Build history of the part. All positions in model axes, mm. Give positions to 0.01 mm unless a question says otherwise; leave off trailing zeros. Order: outer loops, then holes, each group sorted by start corner. A loop starts at its lowest first (then second) coordinate and runs counter-clockwise, first axis right, second up. Notation, with made-up numbers: M -35.5,-6 L -9.5,-6 A9 cw -9.5,1 Z; hole C -10,23 d11. An arc over 180 degrees is marked long. One line per item, written item: value.
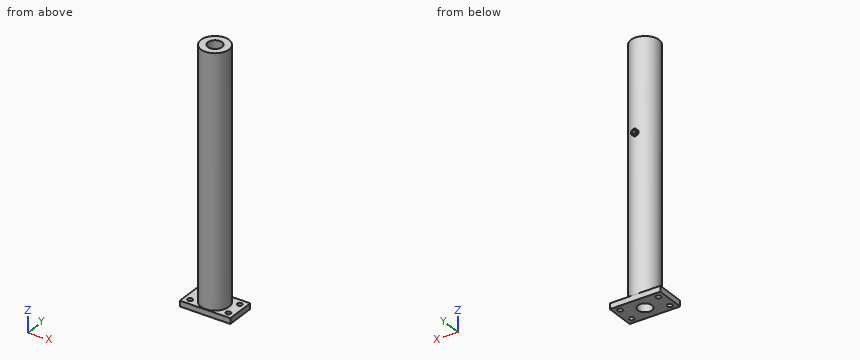
Autodesk Fusion 360 part; units mm, degrees
sketch "Sketch1" plane through (0, 0, 0) normal (0, 0, 1) x (1, 0, 0)
  circle A0 centre (0, 0) radius 6.375
  circle A1 centre (0, 0) radius 12.5
  dimension "d1" = 25
  dimension "d2" = 12.75
extrude "Extrude1" add sketch "Sketch1" along normal blind 225 contours A0 | A1
extrude "Extrude19" cut sketch "Sketch1" along normal up to surface (225 mm away) contours A0
sketch "Sketch22" plane through (0, 0, 0) normal (0, 0, 1) x (1, 0, 0)
  line L0 (22.5, 13) -> (-22.5, 13)
  line L1 (-22.5, 13) -> (-22.5, -13)
  line L2 (-22.5, -13) -> (22.5, -13)
  line L3 (22.5, -13) -> (22.5, 13)
  circle A0 centre (0, 0) radius 6.375 construction
  circle A1 centre (0, 0) radius 12.5 construction
  line L4 (0, 0) -> (22.5, 0) construction
  line L5 (0, 0) -> (-22.5, 0) construction
  circle A2 centre (0, 0) radius 12.5
  circle A3 centre (17, 7.5) radius 2.25
  circle A4 centre (-17, 7.5) radius 2.25
  circle A5 centre (-17, -7.5) radius 2.25
  circle A6 centre (17, -7.5) radius 2.25
  point P0 (12.5, 0)
  point P1 (-12.5, 0)
  dimension "d150" = 10
  dimension "d151" = 10
  dimension "d152" = 13
  dimension "d155" = 4.5
  dimension "d156" = 17
  dimension "d157" = 17
  dimension "d158" = 17
  dimension "d159" = 17
  dimension "d160" = 4.5
  dimension "d161" = 4.5
  dimension "d162" = 4.5
  dimension "d163" = 7.5
  dimension "d164" = 7.5
  dimension "d165" = 7.5
  dimension "d166" = 7.5
extrude "Mount Holes" add sketch "Sketch22" along normal blind 5
ref_plane "WorkPlane4" through (0, 6.4, 0) normal (0, 1, 0) x (0, 0, 1)
sketch "Sketch21" plane through (0, 6.4, 0) normal (0, 1, 0) x (1, 0, 0)
  circle A0 centre (0, -143.363) radius 1.7
  circle A1 centre (0, -143.363) radius 2.7
  line L0 (-12.5, -225) -> (12.5, -225)
  line L1 (22.5, 0) -> (-22.5, 0) construction
  line L2 (-22.5, 0) -> (-22.5, -5) construction
  line L3 (-22.5, -5) -> (22.5, -5) construction
  line L4 (22.5, -5) -> (22.5, 0) construction
  line L5 (0, -5) -> (0, -225) construction
  dimension "d137" = 3.4
  dimension "d138" = 5.4
  dimension "d167" = 81.637
extrude "Extrude17" add sketch "Sketch21" along normal blind 8
extrude "Extrude18" cut sketch "Sketch21" along normal blind 8 and the other way blind 2 contours A0
equation "d22 = d20"
equation "d136 = d5 / 2"
equation "d138 = d137 + 2 mm"
equation "d151 = d150"
equation "d157 = d156"
equation "d158 = d156"
equation "d159 = d156"
equation "d160 = d155"
equation "d161 = d155"
equation "d162 = d155"
equation "d164 = d163"
equation "d165 = d163"
equation "d166 = d163"
1) Drill centre lines: probe 1 along Y at (x, z) = (-17, 2); probe 2 along X at (y, z) = (-0.75, 155); probe 3 along Z at (x, y) = (0, 11). Where is each one in solid material? Low to high. Write a range as from..to.
Check values:
probe 1: -13..-9.75, -5.25..5.25, 9.75..13
probe 2: -12.48..-6.33, 6.33..12.48
probe 3: 0..141.66, 145.06..225
2) Saw through at A-A, the plane x = -17. Write the cut outline in (y, z).
Check values:
outline: M -13,0 L -9.75,0 L -9.75,5 L -13,5 Z; M -5.25,0 L 5.25,0 L 5.25,5 L -5.25,5 Z; M 9.75,0 L 13,0 L 13,5 L 9.75,5 Z
3) Saw through at B-B, the plane z = 57. Write the cut outline in (x, y) (3 decimals), then the cut area to 3 significant figures.
Check values:
outline: C 0,0 d25; hole C 0,0 d12.75
area: 363 mm^2
4) Pin check, flat tips, straight feed: pin 1 (1.5 mm diameter, centred on x = -1, z = 2, fed in from +Y); pin 2 (3 mm diameter, centred on x = 0, z = 143.363, fed in from +Y); pin 3 (6 mm diameter, centred on x = -17, y = -7.5, fed in from +Z); pin 4 (5 mm diameter, centred on x = -17, y = 7.5, fed in from -Z). Stop position of each tip, or through.
Check values:
pin 1: y = 13
pin 2: y = -6.2
pin 3: z = 5
pin 4: z = 0
